Here's how the part is built. I have some questions about the finished solid (model axes, mm). A direction names the side the tool comes from. Round coordinates to 2 decimals unless told otherwise and drop trailing zeros. Put each result on its own line as item: value. Start each with the question number.
1. We'd pull the mould along Z, two halves only. Please class faces 1 (the face through (-26.841, -3, 8)), 2 (the face through (-24.841, -3, 7)), 3 (the face through (-48, -3, 22.247)), 4 (the face through (-40, -3, 1.247)): +Z half, -Z half, draft (parallel to the pull), parting line (faces both ways), or undercut.
2. Which directions (+Z, -Z, +X, -X, +Y, -Y) give clear straight access to the entire face, cutting with the end or side of a thin tool? Please do faces 5 (the face through (-33.841, -3, 7)), 6 (the face through (-40, -225, 11)).
3. I need wall thicknesses on probe 1 along Z at (x, y) = (-43.5, -162); probe 2 along X at (y, z) = (129.5, 8); probe 3 along X at (y, z) = (184, 6). Which ranges of each line are inside material? Lowest first, please. Write a range as from..to.
4. For pin 1 (1.5 mm diameter, centred on x = -40.5, y = -19.5, fed in from +Z); pin 2 (1 mm diameter, centred on x = -38.5, z = 14, fed in from -Y); pin 3 (1.2 mm diameter, centred on y = -106.5, z = 4.5, fed in from -X); pin 4 (4.5 mm diameter, centred on x = -42.5, y = 51, fed in from +Z), each with a flat end and sliding along its axis, tell me the tip position at first contact or that it passes through.
5. Suppose I cut it at A-A (y = 8.5). Count the separate pieces of the cut face and the enclosed holes in it, then the cut area to 3 significant figures.
```python
from build123d import *

# Parameters (mm, degrees)
F2_DEPTH = 225


# Not quite as in the source:
# - ends of sketch curves that miss each other by under 0.0002 mm in the source are joined


with BuildPart() as f2:
    # F1 (on Front) → F2 (new body, symmetric)
    with BuildSketch(Plane.XZ):
        with BuildLine():
            Line((-48.090856, 20.246586), (-44.140856, 20.246586))
            ThreePointArc((-44.140856, 20.246586), (-43.9287239656, 20.3344539656), (-43.840856, 20.546586))
            Line((-43.840856, 20.546586), (-43.840856, 21.946586))
            ThreePointArc((-43.840856, 21.946586), (-43.9287239656, 22.1587180344), (-44.140856, 22.246586))
            Line((-44.140856, 22.246586), (-52.840856, 22.246586))
            ThreePointArc((-52.840856, 22.246586), (-54.2550695624, 21.6607995624), (-54.840856, 20.246586))
            Line((-54.840856, 20.246586), (-54.840856, 11.546586))
            ThreePointArc((-54.840856, 11.546586), (-54.7529880344, 11.3344539656), (-54.540856, 11.246586))
            Line((-54.540856, 11.246586), (-53.140856, 11.246586))
            ThreePointArc((-53.140856, 11.246586), (-52.9287239656, 11.3344539656), (-52.840856, 11.546586))
            Line((-52.840856, 11.546586), (-52.840856, 15.496586))
            Line((-52.840856, 15.496586), (-49.50507, 15.496586))
            Line((-49.50507, 15.496586), (-45.840856, 11.832372))
            Line((-45.840856, 11.832372), (-45.840856, 7.900176))
            ThreePointArc((-45.840856, 7.900176), (-45.8238189324, 7.7707665494), (-45.7738687764, 7.6501761291))
            Line((-45.7738687764, 7.6501761291), (-45.540856, 7.246586))
            Line((-45.540856, 7.246586), (-45.773869, 6.842996))
            ThreePointArc((-45.773869, 6.842996), (-45.840856, 6.592996), (-45.7738687764, 6.3429961291))
            Line((-45.7738687764, 6.3429961291), (-45.591833, 6.0277))
            Line((-45.591833, 6.0277), (-45.840856, 4.746586))
            Line((-45.840856, 4.746586), (-45.840856, 2.6608))
            Line((-45.840856, 2.6608), (-49.50507, -1.003414))
            Line((-49.50507, -1.003414), (-52.840856, -1.003414))
            Line((-52.840856, -1.003414), (-52.840856, 2.946586))
            ThreePointArc((-52.840856, 2.946586), (-52.9287239656, 3.1587180344), (-53.140856, 3.246586))
            Line((-53.140856, 3.246586), (-54.540856, 3.246586))
            ThreePointArc((-54.540856, 3.246586), (-54.7529880344, 3.1587180344), (-54.840856, 2.946586))
            Line((-54.840856, 2.946586), (-54.840856, -5.753414))
            ThreePointArc((-54.840856, -5.753414), (-54.2550695624, -7.1676275624), (-52.840856, -7.753414))
            Line((-52.840856, -7.753414), (-26.840856, -7.753414))
            ThreePointArc((-26.840856, -7.753414), (-25.4266424376, -7.1676275624), (-24.840856, -5.753414))
            Line((-24.840856, -5.753414), (-24.840856, 20.246586))
            ThreePointArc((-24.840856, 20.246586), (-25.4266424376, 21.6607995624), (-26.840856, 22.246586))
            Line((-26.840856, 22.246586), (-35.540856, 22.246586))
            ThreePointArc((-35.540856, 22.246586), (-35.7529880344, 22.1587180344), (-35.840856, 21.946586))
            Line((-35.840856, 21.946586), (-35.840856, 20.546586))
            ThreePointArc((-35.840856, 20.546586), (-35.7529880344, 20.3344539656), (-35.540856, 20.246586))
            Line((-35.540856, 20.246586), (-31.590856, 20.246586))
            Line((-31.590856, 20.246586), (-31.590856, 16.9108))
            Line((-31.590856, 16.9108), (-35.25507, 13.246586))
            Line((-35.25507, 13.246586), (-39.187266, 13.246586))
            ThreePointArc((-39.187266, 13.246586), (-39.3166754506, 13.2295489324), (-39.4372658709, 13.1795987764))
            Line((-39.4372658709, 13.1795987764), (-39.840856, 12.946586))
            Line((-39.840856, 12.946586), (-40.244446, 13.179599))
            ThreePointArc((-40.244446, 13.179599), (-40.494446, 13.246586), (-40.7444458709, 13.1795987764))
            Line((-40.7444458709, 13.1795987764), (-41.059742, 12.997563))
            Line((-41.059742, 12.997563), (-42.340856, 13.246586))
            Line((-42.340856, 13.246586), (-44.426642, 13.246586))
            Line((-44.426642, 13.246586), (-48.090856, 16.9108))
            Line((-48.090856, 16.9108), (-48.090856, 20.246586))
        make_face()
        with BuildLine():
            ThreePointArc((-48.030175, -5.753414), (-48.180175082, -5.7132215738), (-48.2899827159, -5.6034138359))
            ThreePointArc((-48.2899827159, -5.6034138359), (-49.1151948384, -5.1042472042), (-49.9783690315, -5.5344479782))
            ThreePointArc((-49.9783690315, -5.5344479782), (-53.0449723505, -5.6142903949), (-52.1906940253, -2.6679979306))
            Line((-52.1906940253, -2.6679979306), (-50.91426, -2.203414))
            Line((-50.91426, -2.203414), (-48.290856, -2.203414))
            ThreePointArc((-48.290856, -2.203414), (-47.9081725676, -2.1272935325), (-47.5837492188, -1.9105207812))
            Line((-47.5837492188, -1.9105207812), (-44.719536, 0.953693))
            ThreePointArc((-44.719536, 0.953693), (-44.3951124324, 1.1704655325), (-44.012429, 1.246586))
            Line((-44.012429, 1.246586), (-35.669283, 1.246586))
            ThreePointArc((-35.669283, 1.246586), (-35.2865995676, 1.1704655325), (-34.9621762188, 0.9536927812))
            Line((-34.9621762188, 0.9536927812), (-31.883749, -2.124734))
            ThreePointArc((-31.883749, -2.124734), (-31.6669764675, -2.4491575676), (-31.590856, -2.831841))
            Line((-31.590856, -2.831841), (-31.590856, -4.753414))
            ThreePointArc((-31.590856, -4.753414), (-31.8837492188, -5.4605207812), (-32.590856, -5.753414))
            Line((-32.590856, -5.753414), (-48.030175, -5.753414))
        make_face(mode=Mode.SUBTRACT)
        with BuildLine():
            ThreePointArc((-30.2930043339, -4.0956641215), (-29.9673844937, -2.6268855063), (-28.4986058785, -2.3012656661))
            Line((-28.4986058785, -2.3012656661), (-27.491018, -2.667998))
            ThreePointArc((-27.491018, -2.667998), (-26.7973531157, -5.7969168843), (-29.9262720694, -5.1032520253))
            Line((-29.9262720694, -5.1032520253), (-30.2930043339, -4.0956641215))
        make_face(mode=Mode.SUBTRACT)
        with BuildLine():
            ThreePointArc((-36.5876690145, 8.2349049956), (-36.440856, 7.246586), (-36.5876690145, 6.2582670044))
            ThreePointArc((-36.5876690145, 6.2582670044), (-36.5433888407, 5.9288023569), (-36.2653470651, 5.7465855742))
            ThreePointArc((-36.2653470651, 5.7465855742), (-35.9615444769, 5.5780848975), (-35.840856, 5.25232))
            Line((-35.840856, 5.25232), (-35.840856, 3.746586))
            ThreePointArc((-35.840856, 3.746586), (-35.9873026094, 3.3930326094), (-36.340856, 3.246586))
            Line((-36.340856, 3.246586), (-37.84659, 3.246586))
            ThreePointArc((-37.84659, 3.246586), (-38.1723548975, 3.3672744769), (-38.3408555178, 3.6710770737))
            ThreePointArc((-38.3408555178, 3.6710770737), (-38.5230723569, 3.9491188407), (-38.8525409519, 3.9933978415))
            ThreePointArc((-38.8525409519, 3.9933978415), (-39.840856, 3.846586), (-40.8291749956, 3.9933990145))
            ThreePointArc((-40.8291749956, 3.9933990145), (-41.1586396431, 3.9491188407), (-41.3408564258, 3.6710770651))
            ThreePointArc((-41.3408564258, 3.6710770651), (-41.5093571025, 3.3672744769), (-41.835122, 3.246586))
            Line((-41.835122, 3.246586), (-43.340856, 3.246586))
            ThreePointArc((-43.340856, 3.246586), (-43.6944093906, 3.3930326094), (-43.840856, 3.746586))
            Line((-43.840856, 3.746586), (-43.840856, 5.25232))
            ThreePointArc((-43.840856, 5.25232), (-43.7201675231, 5.5780848975), (-43.4163649263, 5.7465855178))
            ThreePointArc((-43.4163649263, 5.7465855178), (-43.1383231593, 5.9288023569), (-43.0940441585, 6.2582709519))
            ThreePointArc((-43.0940441585, 6.2582709519), (-43.240856, 7.246586), (-43.0940429855, 8.2349049956))
            ThreePointArc((-43.0940429855, 8.2349049956), (-43.1383231593, 8.5643696431), (-43.4163649349, 8.7465864258))
            ThreePointArc((-43.4163649349, 8.7465864258), (-43.7201675231, 8.9150871025), (-43.840856, 9.240852))
            Line((-43.840856, 9.240852), (-43.840856, 10.746586))
            ThreePointArc((-43.840856, 10.746586), (-43.6944093906, 11.1001393906), (-43.340856, 11.246586))
            Line((-43.340856, 11.246586), (-41.835122, 11.246586))
            ThreePointArc((-41.835122, 11.246586), (-41.5093571025, 11.1258975231), (-41.3408564822, 10.8220949263))
            ThreePointArc((-41.3408564822, 10.8220949263), (-41.1586396431, 10.5440531593), (-40.8291710481, 10.4997741585))
            ThreePointArc((-40.8291710481, 10.4997741585), (-39.840856, 10.646586), (-38.8525370044, 10.4997729855))
            ThreePointArc((-38.8525370044, 10.4997729855), (-38.5230723569, 10.5440531593), (-38.3408555742, 10.8220949349))
            ThreePointArc((-38.3408555742, 10.8220949349), (-38.1723548975, 11.1258975231), (-37.84659, 11.246586))
            Line((-37.84659, 11.246586), (-36.340856, 11.246586))
            ThreePointArc((-36.340856, 11.246586), (-35.9873026094, 11.1001393906), (-35.840856, 10.746586))
            Line((-35.840856, 10.746586), (-35.840856, 9.240852))
            ThreePointArc((-35.840856, 9.240852), (-35.9615444769, 8.9150871025), (-36.2653470737, 8.7465864822))
            ThreePointArc((-36.2653470737, 8.7465864822), (-36.5433888407, 8.5643696431), (-36.5876690145, 8.2349049956))
        make_face(mode=Mode.SUBTRACT)
        with BuildLine():
            ThreePointArc((-49.3887076661, 18.5888361215), (-49.7143275063, 17.1200575063), (-51.1831061215, 16.7944376661))
            Line((-51.1831061215, 16.7944376661), (-52.190694, 17.16117))
            ThreePointArc((-52.190694, 17.16117), (-52.8843588843, 20.2900888843), (-49.7554399306, 19.5964240253))
            Line((-49.7554399306, 19.5964240253), (-49.3887076661, 18.5888361215))
        make_face(mode=Mode.SUBTRACT)
        with BuildLine():
            ThreePointArc((-33.5479627812, 2.3679062188), (-33.7647355325, 2.6923295676), (-33.840856, 3.075013))
            Line((-33.840856, 3.075013), (-33.840856, 11.418159))
            ThreePointArc((-33.840856, 11.418159), (-33.7647355325, 11.8008424324), (-33.5479627812, 12.1252657812))
            Line((-33.5479627812, 12.1252657812), (-30.683749, 14.989479))
            ThreePointArc((-30.683749, 14.989479), (-30.4669764675, 15.3139025676), (-30.390856, 15.696586))
            Line((-30.390856, 15.696586), (-30.390856, 18.31999))
            Line((-30.390856, 18.31999), (-29.926272, 19.596424))
            ThreePointArc((-29.926272, 19.596424), (-26.9799796051, 20.4507023505), (-27.0598220201, 17.3840990291))
            ThreePointArc((-27.0598220201, 17.3840990291), (-27.4900227958, 16.5209248384), (-26.9908561748, 15.6957126972))
            ThreePointArc((-26.9908561748, 15.6957126972), (-26.8810484262, 15.585905082), (-26.840856, 15.435905))
            Line((-26.840856, 15.435905), (-26.840856, -0.003414))
            ThreePointArc((-26.840856, -0.003414), (-27.1337492188, -0.7105207812), (-27.840856, -1.003414))
            Line((-27.840856, -1.003414), (-29.762429, -1.003414))
            ThreePointArc((-29.762429, -1.003414), (-30.1451124324, -0.9272935325), (-30.4695357812, -0.7105207812))
            Line((-30.4695357812, -0.7105207812), (-33.5479627812, 2.3679062188))
        make_face(mode=Mode.SUBTRACT)
    extrude(amount=F2_DEPTH, both=True)


solid = f2.part
```
Verdict:
1. face 1: undercut
1. face 2: draft
1. face 3: +Z half
1. face 4: undercut
2. face 5: +Y, -Y
2. face 6: +Z, -Z, +X, -X, -Y
3. probe 1: z = -7.75..-5.75, 1.25..3.27, 5.73..8.77, 11.22..13.25
3. probe 2: x = -45.84..-43.16, -36.53..-33.84, -26.84..-24.84
3. probe 3: x = -45.6..-43.1, -36.58..-33.84, -26.84..-24.84
4. pin 1: stops at z = 13.25
4. pin 2: passes through
4. pin 3: stops at x = -45.84
4. pin 4: stops at z = 22.25
5. separate pieces: 1
5. enclosed holes: 5
5. area: 339 mm^2
